```python
from build123d import *

# Parameters (mm, degrees)
F1_DEPTH   = 60
F2_R       = 2.5
F3_DEPTH   = 5.001
F4_R       = 1
F1_FACE1_R = 10
F5_DEPTH   = 25


with BuildPart() as f1:
    # F0 (on Front) → F1 (new body)
    with BuildSketch(Plane.XZ):
        with BuildLine():
            Line((69.3844701811, 66.6805505753), (86.5065387851, 108.4481678561))
            ThreePointArc((86.5065387851, 108.4481678561), (92.0400214246, 102.28627745), (100, 100))
            Line((100, 100), (100, 105))
            ThreePointArc((100, 105), (92.9289321881, 107.9289321881), (90, 115))
            Line((90, 115), (83.7885603577, 115))
            Line((83.7885603577, 115), (63.980656967, 66.6805505753))
            Line((63.980656967, 66.6805505753), (69.3844701811, 66.6805505753))
        make_face()
        with BuildLine():
            Line((100, 105), (100, 100))
            ThreePointArc((100, 100), (107.9599785754, 102.28627745), (113.4934612149, 108.4481678561))
            Line((113.4934612149, 108.4481678561), (141.5528599106, 40))
            Line((141.5528599106, 40), (58.4471400894, 40))
            Line((58.4471400894, 40), (69.3844701811, 66.6805505753))
            Line((69.3844701811, 66.6805505753), (63.980656967, 66.6805505753))
            Line((63.980656967, 66.6805505753), (36.6458690181, 0))
            Line((36.6458690181, 0), (0, 0))
            Line((0, 0), (0, -5))
            Line((0, -5), (40, -5))
            Line((40, -5), (56.3974578573, 35))
            Line((56.3974578573, 35), (143.6025421427, 35))
            Line((143.6025421427, 35), (160, -5))
            Line((160, -5), (200, -5))
            Line((200, -5), (200, 0))
            Line((200, 0), (163.3541309819, 0))
            Line((163.3541309819, 0), (113.8790881603, 120.6895440801))
            ThreePointArc((113.8790881603, 120.6895440801), (100, 130), (86.1209118397, 120.6895440801))
            Line((86.1209118397, 120.6895440801), (83.7885603577, 115))
            Line((83.7885603577, 115), (90, 115))
            ThreePointArc((90, 115), (100, 125), (110, 115))
            ThreePointArc((110, 115), (107.0710678119, 107.9289321881), (100, 105))
        make_face()
        Polygon((43.611112982, 66.6805505753), (63.980656967, 66.6805505753), (83.7885603577, 115), (43.611112982, 115), align=None)
    extrude(amount=-F1_DEPTH)

    # F2 (on face) → F3 (cut, through all)
    with BuildSketch(Plane.XY):
        with Locations((182.5, 10)):
            Circle(F2_R)
        with Locations((182.5, 42.5)):
            Circle(F2_R)
        with Locations((17.5, 10)):
            Circle(F2_R)
        with Locations((17.5, 42.5)):
            Circle(F2_R)
    extrude(amount=-F3_DEPTH, mode=Mode.SUBTRACT)

    # F4
    f4_edges = [f1.edges().sort_by_distance(p)[0] for p in [
        (200, 30, 0),
        (200, 30, -5),
        (0, 30, 0),
        (0, 30, -5),
        (151.801271, 0, 15),
        (180, 0, -5),
        (20, 0, -5),
        (48.198729, 0, 15),
    ]]
    fillet(f4_edges, radius=F4_R)

    # F0 (on Front) + F1_face1 (on face) → F5 (join)
    with BuildSketch(Plane.XZ):
        with BuildLine():
            Line((69.3844701811, 66.6805505753), (86.5065387851, 108.4481678561))
            ThreePointArc((86.5065387851, 108.4481678561), (92.0400214246, 102.28627745), (100, 100))
            Line((100, 100), (100, 105))
            ThreePointArc((100, 105), (92.9289321881, 107.9289321881), (90, 115))
            Line((90, 115), (83.7885603577, 115))
            Line((83.7885603577, 115), (63.980656967, 66.6805505753))
            Line((63.980656967, 66.6805505753), (69.3844701811, 66.6805505753))
        make_face()
        with BuildLine():
            Line((100, 105), (100, 100))
            ThreePointArc((100, 100), (107.9599785754, 102.28627745), (113.4934612149, 108.4481678561))
            Line((113.4934612149, 108.4481678561), (141.5528599106, 40))
            Line((141.5528599106, 40), (58.4471400894, 40))
            Line((58.4471400894, 40), (69.3844701811, 66.6805505753))
            Line((69.3844701811, 66.6805505753), (63.980656967, 66.6805505753))
            Line((63.980656967, 66.6805505753), (36.6458690181, 0))
            Line((36.6458690181, 0), (0, 0))
            Line((0, 0), (0, -5))
            Line((0, -5), (40, -5))
            Line((40, -5), (56.3974578573, 35))
            Line((56.3974578573, 35), (143.6025421427, 35))
            Line((143.6025421427, 35), (160, -5))
            Line((160, -5), (200, -5))
            Line((200, -5), (200, 0))
            Line((200, 0), (163.3541309819, 0))
            Line((163.3541309819, 0), (113.8790881603, 120.6895440801))
            ThreePointArc((113.8790881603, 120.6895440801), (100, 130), (86.1209118397, 120.6895440801))
            Line((86.1209118397, 120.6895440801), (83.7885603577, 115))
            Line((83.7885603577, 115), (90, 115))
            ThreePointArc((90, 115), (100, 125), (110, 115))
            ThreePointArc((110, 115), (107.0710678119, 107.9289321881), (100, 105))
        make_face()
        Polygon((43.611112982, 66.6805505753), (63.980656967, 66.6805505753), (83.7885603577, 115), (43.611112982, 115), align=None)
    with BuildSketch(Plane(origin=(84.7585463742, 60, 67.9155553521), x_dir=(1, 0, 0), z_dir=(0, 1, 0))):
        with BuildLine():
            Line((-83.7585463742, 67.9155553521), (-48.1126773562, 67.9155553521))
            Line((-48.1126773562, 67.9155553521), (-20.7778894072, 1.2350047768))
            Line((-20.7778894072, 1.2350047768), (-41.1474333922, 1.2350047768))
            Line((-41.1474333922, 1.2350047768), (-41.1474333922, -47.0844446479))
            Line((-41.1474333922, -47.0844446479), (-0.9699860165, -47.0844446479))
            Line((-0.9699860165, -47.0844446479), (1.3623654655, -52.7739887281))
            ThreePointArc((1.3623654655, -52.7739887281), (15.2414536258, -62.0844446479), (29.120541786, -52.7739887281))
            Line((29.120541786, -52.7739887281), (78.5955846077, 67.9155553521))
            Line((78.5955846077, 67.9155553521), (114.2414536258, 67.9155553521))
            ThreePointArc((114.2414536258, 67.9155553521), (114.948560407, 68.2084485709), (115.2414536258, 68.9155553521))
            Line((115.2414536258, 68.9155553521), (115.2414536258, 71.9155553521))
            ThreePointArc((115.2414536258, 71.9155553521), (114.948560407, 72.6226621332), (114.2414536258, 72.9155553521))
            Line((114.2414536258, 72.9155553521), (75.2414536258, 72.9155553521))
            Line((75.2414536258, 72.9155553521), (58.8439957685, 32.9155553521))
            Line((58.8439957685, 32.9155553521), (-28.3610885169, 32.9155553521))
            Line((-28.3610885169, 32.9155553521), (-44.7585463742, 72.9155553521))
            Line((-44.7585463742, 72.9155553521), (-83.7585463742, 72.9155553521))
            ThreePointArc((-83.7585463742, 72.9155553521), (-84.4656531554, 72.6226621332), (-84.7585463742, 71.9155553521))
            Line((-84.7585463742, 71.9155553521), (-84.7585463742, 68.9155553521))
            ThreePointArc((-84.7585463742, 68.9155553521), (-84.4656531554, 68.2084485709), (-83.7585463742, 67.9155553521))
        make_face()
        with BuildLine():
            ThreePointArc((28.7349148407, -40.532612504), (15.2414536258, -32.0844446479), (1.7479924109, -40.532612504))
            Line((1.7479924109, -40.532612504), (-26.3114062848, 27.9155553521))
            Line((-26.3114062848, 27.9155553521), (56.7943135364, 27.9155553521))
            Line((56.7943135364, 27.9155553521), (28.7349148407, -40.532612504))
        make_face(mode=Mode.SUBTRACT)
        with Locations((15.2414536258, -47.0844446479)):
            Circle(F1_FACE1_R, mode=Mode.SUBTRACT)
    extrude(amount=F5_DEPTH, dir=(0, -1, 0))


solid = f1.part
```
Geometry check sheet. Reference: the model listing, model coordinates, mm. A direction names the side the tool comes from. Coordinates: 2 decimals unless noted, no trailing zeros. Write each loop counter-clockwise with the first axis right and the second up, starting at its lowest first coordinate (ties: lowest second). Pieces come first, ordered by that corner, then holes. Notation, with made-up numbers: (21, 67) -> (64, 67) arc R22 ccw to (64, 100) -> close; hole circle Ø5 at (1.25, 0.25). An arc over 180 degrees is marked (long way). Use CSV: the item, a comma, the result in double quotes. Start each with the question number.
Item 1: Cross-section at B-B, the plane z = 44. Record the cut outline in (x, y).
Item 2: Thickness scan on line 1 (Y direction, x = 182.5, z = -1.4); line 2 (X direction, y = -20, z = 106); line 3 (Y direction, x = 17, z = -1). Record the ranges inside material, lowest first.
Item 3: Depth check by flat-ended pin: pin 1 Ø10.5 at (x, y) = (26, 17.5) entering from +Z; pin 2 Ø12.5 at (x, y) = (88, 51) entering from -Z; pin 3 Ø6 at (x, z) = (145.5, 59) entering from +Y; pin 4 Ø10 at (x, y) = (52.5, -18.5) entering from -Z. Enter the tip coordinate at first touch or a pass-through.
Item 4: Cross-section at C-C, the plane y = 28.5. Record the cut outline in (x, z).
Item 5: Mould release check, pull along Z, two halves, no side actions. Record for faces 1 (the cylindrical face through (16, 8, -2)), 2 (the flat face through (20, -12, -5)), 3 (the flat face through (72.28, 18.1, 73.74)): released by +Z, released by -Z, zero draft, split by the parting line, or undercut.
Item 6: Cross-section at D-D, the plane y = 10. State how many separate pieces and enclosed holes the cut face has, plus the area to 3 significant figures.
Item 7: Set-up check for faces 4 (the flat face through (70, -25, 78)), 5 (the flat face through (101, 18, 40)), 6 (the flat face through (151.686, -12.325, 15.28)): record each of +Z, -Z, +X, -X, +Y, -Y from which the full face is reachable in a straight line by a thin tool's end or side.
Item 8: Cross-section at A-A, the plane x = 182.5. Record the cut outline in (y, z).
Answers:
1,outline,"(54.68, -25) -> (60.09, -25) -> (60.09, 60) -> (54.68, 60) -> close; (139.91, -25) -> (145.32, -25) -> (145.32, 60) -> (139.91, 60) -> close"
2,line 1,"-25 to 7.5, 12.5 to 60"
2,line 2,"43.61 to 85.5, 88 to 95.64, 104.36 to 112, 114.5 to 119.9"
2,line 3,"-25 to 7.55, 12.45 to 60"
3,pin 1,"z = 0"
3,pin 2,"z = 35"
3,pin 3,"through"
3,pin 4,"z = 13.3"
4,outline,"(0, -4) arc R1 ccw to (1, -5) -> (40, -5) -> (56.4, 35) -> (143.6, 35) -> (160, -5) -> (199, -5) arc R1 ccw to (200, -4) -> (200, -1) arc R1 ccw to (199, 0) -> (163.35, 0) -> (113.88, 120.69) arc R15 ccw to (86.12, 120.69) -> (83.79, 115) -> (43.61, 115) -> (43.61, 66.68) -> (63.98, 66.68) -> (36.65, 0) -> (1, 0) arc R1 ccw to (0, -1) -> close; hole (58.45, 40) -> (141.55, 40) -> (113.49, 108.45) arc R15 cw to (86.51, 108.45) -> close; hole circle Ø20 at (100, 115)"
5,face 1,"zero draft"
5,face 2,"released by -Z"
5,face 3,"undercut"
6,separate pieces,"3"
6,enclosed holes,"2"
6,area,"3,860 mm^2"
7,face 4,"+Z, -Z, +X, -X, -Y"
7,face 5,"+Y, -Y"
7,face 6,"-Z, +Y, -Y"
8,outline,"(-25, -5) -> (0, -5) -> (0, -4) arc R1 ccw to (1, -5) -> (7.5, -5) -> (7.5, 0) -> (-25, 0) -> close; (12.5, -5) -> (60, -5) -> (60, 0) -> (12.5, 0) -> close"
